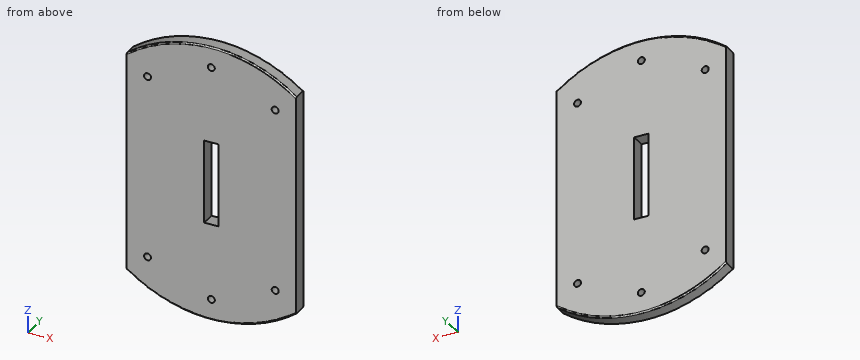
Autodesk Inventor part; units mm, degrees
ref_plane "YZ Plane" through (0, 0, 0) normal (1, 0, 0) x (0, 1, 0)
ref_plane "XZ Plane" through (0, 0, 0) normal (0, 1, 0) x (-1, 0, 0)
ref_plane "XY Plane" through (0, 0, 0) normal (0, 0, 1) x (1, 0, 0)
sketch "Sketch1" plane through (0, 0, 0) normal (0, 1, 0) x (-1, 0, 0)
  circle A0 centre (0, 0) radius 50
  line L0 (-25.38, 0) -> (-25.38, 35.55)
  line L1 (-25.38, 35.55) -> (0, 35.55)
  line L2 (25.38, 35.55) -> (0, 35.55)
  line L3 (25.38, 35.55) -> (25.38, 0)
  line L4 (-25.38, 0) -> (-25.38, -35.55)
  line L5 (-25.38, -35.55) -> (0, -35.55)
  line L6 (25.38, -35.55) -> (0, -35.55)
  line L7 (25.38, -35.55) -> (25.38, 0)
  line L8 (-25.38, -35.55) -> (-25.38, -33.05)
  line L9 (-25.38, -33.05) -> (-22.88, -33.05)
  circle A1 centre (-22.88, -33.05) radius 1.25
  line L10 (-25.38, 35.55) -> (-25.38, 33.05)
  line L11 (-25.38, 33.05) -> (-22.88, 33.05)
  circle A2 centre (-22.88, 33.05) radius 1.25
  line L12 (25.38, 35.55) -> (25.38, 33.05)
  line L13 (25.38, 33.05) -> (22.88, 33.05)
  circle A3 centre (22.88, 33.05) radius 1.25
  line L14 (25.38, -35.55) -> (25.38, -33.05)
  line L15 (25.38, -33.05) -> (22.88, -33.05)
  circle A4 centre (22.88, -33.05) radius 1.25
  dimension "d0" = 100
  dimension "d4" = 50.76
  dimension "d5" = 2.5
  dimension "d6" = 2.5
  dimension "d7" = 2.5
  dimension "d8" = 2.5
  dimension "d9" = 2.5
  dimension "d10" = 2.5
  dimension "d11" = 2.5
  dimension "d12" = 2.5
  dimension "d13" = 2.5
  dimension "d14" = 2.5
  dimension "d15" = 2.5
  dimension "d16" = 2.5
extrude "Extrusion1" add sketch "Sketch1" along normal blind 5 contours A0 | L0 L1 L2 L3 L7 L6 L5 L4
sketch "Sketch2" plane through (0, 5, 0) normal (0, 1, 0) x (1, 0, 0)
  line L0 (0, 0) -> (-2.55, 0)
  line L1 (-2.55, 0) -> (2.55, 0)
  line L2 (2.55, 0) -> (2.55, -15.05)
  line L3 (2.55, -15.05) -> (2.55, 15.05)
  line L4 (2.55, 15.05) -> (-2.55, 15.05)
  line L5 (-2.55, 15.05) -> (-2.55, -15.05)
  line L6 (-2.55, -15.05) -> (2.55, -15.05)
  dimension "d19" = 2.55
  dimension "d20" = 5.1
  dimension "d21" = 15.05
  dimension "d22" = 30.1
extrude "Extrusion2" cut sketch "Sketch2" against normal blind 5
sketch "Sketch3" plane through (0, 5, 0) normal (0, 1, 0) x (1, 0, 0)
  circle A0 centre (-22.88, -33.05) radius 1.25
  line L0 (-22.88, -33.05) -> (-30.38, -33.05)
  line L1 (-30.38, -33.05) -> (-30.38, -39.7122)
  circle A1 centre (0, 0) radius 50
  line L2 (-30.38, -33.05) -> (-30.38, 39.7122)
  circle A2 centre (22.88, 33.05) radius 1.25
  line L3 (22.88, 33.05) -> (30.38, 33.05)
  line L4 (30.38, 33.05) -> (30.38, 39.7122)
  line L5 (30.38, 39.7122) -> (30.38, -39.7122)
  dimension "d25" = 7.5
  dimension "d26" = 7.5
extrude "Extrusion3" cut sketch "Sketch3" against normal blind 5 contours L1 A1 L2 | L5 L4 A1
sketch "Sketch4" plane through (0, 5, 0) normal (0, 1, 0) x (1, 0, 0)
  arc A0 (-30.38, -39.7122) -> (30.38, -39.7122) centre (0, 0) ccw
  line L0 (0, -50) -> (0, -42.5)
  circle A1 centre (0, -42.5) radius 1.25
  arc A2 (30.38, 39.7122) -> (-30.38, 39.7122) centre (0, 0) ccw
  line L1 (0, 50) -> (0, 42.5)
  circle A3 centre (0, 42.5) radius 1.25
  dimension "d29" = 7.5
  dimension "d30" = 2.5
  dimension "d31" = 7.5
  dimension "d32" = 2.5
extrude "Extrusion4" cut sketch "Sketch4" against normal blind 5
fillet "Fillet1" radius 0.5 4 edges at (0, 5, 50) (0, 5, -50) (0, 0, 50) (0, 0, -50)
properties part number "Chasis_Cap"
The listing builds one solid part. Answer for the finished solid, in the listing's coordinates (mm). Coordinates: 2 decimals unless noted, no trailing zeros. Write each loop counter-clockwise with the first axis right and the second up, starting at its lowest first coordinate (ties: lowest second). Pieces come first, ordered by that corner, then holes. Notation, with made-up numbers: M 56,-32 L 78,-32 A10 ccw 78,-22 Z; hole C 4.5,34 d5. An arc over 180 degrees is marked long. Put each result on its own line as item: value. Start each with the question number.
1. Flat-ended cylindrical pins translate along their axes: P1, Ø3, axis at x = 0, z = -42.5, coming from the +Y side; P2, Ø2, axis at x = -22.88, z = 33.05, coming from the +Y side; P3, Ø2, axis at x = 19, y = 2.5, coming from the -Z side; P4, Ø2, axis at x = -22, y = 3.5, coming from the -Z side. Find the tip coordinate at first contact, or state that the pin passes through.
2. A cutting plane is placed at A-A on z = -33.05. Write down the section's boundary in (x, y), then the cut area to 3 significant figures.
3. A cutting plane is placed at D-D on x = 22.88. Count the separate pieces of the cut face and the enclosed holes in it, then the cut area to 3 significant figures.
4. A cutting plane is placed at B-B on y = 2.8. Write down the section's boundary in (x, z), then the cut area to 3 significant figures.
5. A cutting plane is placed at C-C on z = 1. Write down the section's boundary in (x, y), then the cut area to 3 significant figures.
6. Consider line 1 (Z direction, x = -1.5, y = 3.1); line 2 (Z direction, x = 22.88, y = 2.05); line 3 (X direction, y = 4.65, z = 11.5). Determine where each line is inside the solid, lowest interval first. Write a range as from..to.
Resolved:
1. P1: stops at y = 5
1. P2: passes through
1. P3: stops at z = -46.65
1. P4: stops at z = -45.38
2. outline: M -30.38,0 L -24.13,0 L -24.13,5 L -30.38,5 Z; M -21.63,0 L 21.63,0 L 21.63,5 L -21.63,5 Z; M 24.13,0 L 30.38,0 L 30.38,5 L 24.13,5 Z
2. area: 279 mm2
3. separate pieces: 3
3. enclosed holes: 0
3. area: 419 mm2
4. outline: M -30.38,-39.71 A50 ccw 30.38,-39.71 L 30.38,39.71 A50 ccw -30.38,39.71 Z; hole C -22.88,-33.05 d2.5; hole C -22.88,33.05 d2.5; hole M -2.55,-15.05 L 2.55,-15.05 L 2.55,15.05 L -2.55,15.05 Z; hole C 0,-42.5 d2.5; hole C 0,42.5 d2.5; hole C 22.88,-33.05 d2.5; hole C 22.88,33.05 d2.5
4. area: 5,500 mm2
5. outline: M -30.38,0 L -2.55,0 L -2.55,5 L -30.38,5 Z; M 2.55,0 L 30.38,0 L 30.38,5 L 2.55,5 Z
5. area: 278 mm2
6. line 1: z = -49.98..-15.05, 15.05..49.98
6. line 2: z = -44.46..-34.3, -31.8..31.8, 34.3..44.46
6. line 3: x = -30.38..-2.55, 2.55..30.38
